CAD build for the part. Positions are in the model's coordinates, mm. Face numbers are marked on the shaded views. Coordinates: 2 decimals unless noted, no trailing zeros. Order: outer loops, then holes, each group sorted by start corner. A loop starts at its lowest first (then second) coordinate and runs counter-clockwise, first axis right, second up. Notation, with made-up numbers: M 52,40.25 L 64,40.25 A20 cw 64,77.25 Z; hole C 16.25,22.5 d2. An arc over 180 degrees is marked long. Write item = value, one per line.
from build123d import *

# Parameters (mm, degrees)
CYLINDER007_R     = 2.6
CYLINDER007_DEPTH = 15
CYLINDER008_R     = 1.6
CYLINDER008_DEPTH = 15
BOX007_W          = 16
BOX007_H          = 40
BOX007_DEPTH      = 13
FILLET_R          = 7
CHAMFER008_SIZE   = 0.4


with BuildPart() as cylinder007:
    # Cylinder007 → Cylinder007 (new body)
    with BuildSketch(Plane(origin=(10, 10, -20), x_dir=(1, 0, 0), z_dir=(0, 0, 1))):
        Circle(CYLINDER007_R)
    extrude(amount=CYLINDER007_DEPTH)


with BuildPart() as fusion009:
    # Cylinder008 → Cylinder008 (new body)
    with BuildSketch(Plane(origin=(10, -20, -20), x_dir=(1, 0, 0), z_dir=(0, 0, 1))):
        Circle(CYLINDER008_R)
    extrude(amount=CYLINDER008_DEPTH)

    # Fusion009: union Cylinder007
    add(cylinder007.part)


with BuildPart() as obj1:
    # Box007 → Box007 (new body)
    with BuildSketch(Plane(origin=(2, -25, -20), x_dir=(1, 0, 0), z_dir=(0, 0, 1))):
        with Locations((8, 20)):
            Rectangle(BOX007_W, BOX007_H)
    extrude(amount=BOX007_DEPTH)

    # Fillet
    fillet_edges = [obj1.edges().sort_by_distance(p)[0] for p in [
        (2, -25, -13.5),
        (2, 15, -13.5),
        (18, -25, -13.5),
        (18, 15, -13.5),
    ]]
    fillet(fillet_edges, radius=FILLET_R)

    # Chamfer008
    chamfer008_edges = [obj1.edges().sort_by_distance(p)[0] for p in [
        (2, -5, -7),
        (2, -5, -20),
        (4.050253, -22.949747, -7),
        (4.050253, 12.949747, -7),
        (10, -25, -7),
        (10, 15, -7),
        (15.949747, -22.949747, -7),
        (15.949747, 12.949747, -7),
        (18, -5, -7),
        (4.050253, -22.949747, -20),
        (4.050253, 12.949747, -20),
        (10, -25, -20),
        (10, 15, -20),
        (15.949747, -22.949747, -20),
        (15.949747, 12.949747, -20),
        (18, -5, -20),
    ]]
    chamfer(chamfer008_edges, length=CHAMFER008_SIZE)

    # Cut008: cut Fusion009
    add(fusion009.part, mode=Mode.SUBTRACT)


with BuildPart() as obj1_1:
    # Cut008 placement: moved
    add(obj1.part.moved(Location((4, 0, 0))))


solid = obj1_1.part
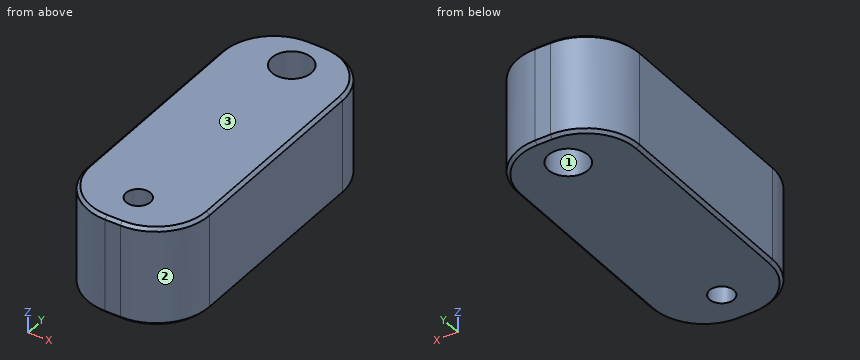
(1) Pull direction X, two halves, no side cores. Call the marked faces 1, 2 and 3: +X half, -X half, draft (parallel to the pull), parting line (faces both ways), or undercut.
Evaluation:
face_1 = undercut
face_2 = +X half
face_3 = draft
(2) Wall check: line 1 (Y direction, x = 14, z = -13); line 2 (Y direction, x = 14.75, z = -14.5); line 3 (X direction, y = 10, z = -15). Give the ranges that are in metal, low to high. Write a range as from..to.
Evaluation:
line_1 = -25..-21.6, -18.4..7.4, 12.6..15
line_2 = -25..-21.41, -18.59..7.51, 12.49..15
line_3 = 6.29..11.4, 16.6..21.71
(3) Slice it at B-B, the plane x = 14. Write the cut outline in (y, z).
Evaluation:
outline = M -25,-19.6 L -24.6,-20 L -21.6,-20 L -21.6,-7 L -24.6,-7 L -25,-7.4 Z; M -18.4,-20 L 7.4,-20 L 7.4,-7 L -18.4,-7 Z; M 12.6,-20 L 14.6,-20 L 15,-19.6 L 15,-7.4 L 14.6,-7 L 12.6,-7 Z
(4) Pin check, flat tips, straight feed: pin 1 Ø2 at (x, z) = (10.5, -17) entering from -Y; pin 2 Ø6 at (x, z) = (19, -9.5) entering from +Y. Stop position of each tip, or through.
Evaluation:
pin_1 = -24.84
pin_2 = 14.93
(5) Slice it at A-A, the plane z = -14. Write the cut outline in (x, y), then the cut area to 3 significant figures.
Evaluation:
outline = M 6,-18 A7 ccw 13,-25 L 15,-25 A7 ccw 22,-18 L 22,8 A7 ccw 15,15 L 13,15 A7 ccw 6,8 Z; hole C 14,10 d5.2; hole C 14,-20 d3.2
area = 569 mm²
